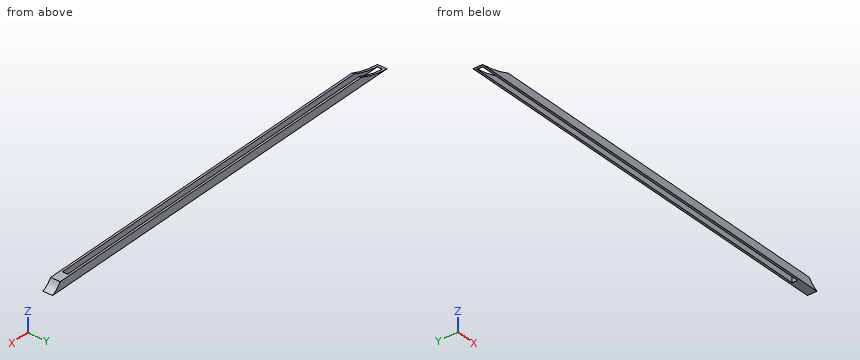
from build123d import *

# Parameters (mm, degrees)
SKETCH1_W               = 512.407402158
SKETCH1_H               = 11.43
SKETCH1_W_2             = 461.607402158
SKETCH1_H_2             = 6.35
BOSS_EXTRUDE1_DEPTH     = 9.652
CUT_EXTRUDE1_DEPTH      = 257.640102966
CUT_EXTRUDE1_DEPTH_BACK = 257.640102966
SKETCH2_R               = 121.331498574
SKETCH2_R_2             = 26.533992322


with BuildPart() as part:
    # Sketch1 → Boss-Extrude1 (new body)
    with BuildSketch(Plane.XY):
        Rectangle(SKETCH1_W, SKETCH1_H)
        Rectangle(SKETCH1_W_2, SKETCH1_H_2, mode=Mode.SUBTRACT)
    extrude(amount=BOSS_EXTRUDE1_DEPTH)

    # Sketch2 → Cut-Extrude1 (cut, two sides: drawn at the far end of the back side and taken through both)
    with BuildSketch(Plane(origin=(0, 5.715, 0), x_dir=(1, 0, 0), z_dir=(0, 1, 0)).offset(-CUT_EXTRUDE1_DEPTH_BACK)):
        with Locations((-245.184147657, -120.830054161)):
            Circle(SKETCH2_R)
        with Locations((267.338172934, -24.084772887)):
            Circle(SKETCH2_R_2)
    extrude(amount=CUT_EXTRUDE1_DEPTH + CUT_EXTRUDE1_DEPTH_BACK, mode=Mode.SUBTRACT)


solid = part.part
Verification items for the finished model (mm, model axes). Round coordinates to 2 decimals unless told otherwise and drop trailing zeros. Loops run counter-clockwise (first coordinate to the right, second up) from the corner with the lowest first, then second, coordinate; pieces in that order, holes last. Notation, with made-up numbers: (30.5, 51.5) - (57.5, 51.5) arc R21 cw to (57.5, 87.5) - close; hole circle Ø4 at (76, -17.5). An arc over 180 degrees is marked (long way). Answer in a Markdown table with one row per item. Add a question column.
Q1. Section check B-B on x = 209. Enter the section's corners in (y, z) (3 decimals).
Q2. Material ranges on line 1 (Y direction, x = 218, z = 5.75) (3 decimals); line 2 (X direction, y = 2, z = 6.75); line 3 (X direction, y = 0, z = 8.75), recorded low to high.
Q3. Section check A-A on y = 1.25. Enter the section's corners in (x, z), plus the area to 3 significant figures.
Q4. Section check C-C on z = 6.5. Enter the section's corners in (x, y) (3 decimals), plus the area to 3 significant figures.
Q5. Gauge pin test, flat ends, axial feed: pin 1 (5 mm diameter, centred on y = -0.5, z = 3, fed in from -X); pin 2 (5 mm diameter, centred on x = 167.5, y = 4.5, fed in from -Z); pin 3 (4 mm diameter, centred on x = -2.5, y = 1, fed in from +Z). Record the tip position at first contact, or that the pin passes through.
Found:
| question | item | result |
|---|---|---|
| 1 | outline | (-5.715, 0) - (-3.175, 0) - (-3.175, 9.652) - (-5.715, 9.652) - close; (3.175, 0) - (5.715, 0) - (5.715, 9.652) - (3.175, 9.652) - close |
| 2 | line 1 | y = -5.715 to -3.175, 3.175 to 5.715 |
| 2 | line 2 | x = 230.8 to 247.25 |
| 2 | line 3 | x = 230.8 to 245.68 |
| 3 | outline | (-234.16, 0) - (-230.8, 0) - (-230.8, 0.35) arc R121.33 cw to start; (230.8, 0) - (256.2, 0) arc R26.53 cw to (245.07, 9.65) - (230.8, 9.65) - close |
| 3 | area | 182 mm² |
| 4 | outline | (-204.564, -5.715) - (247.468, -5.715) - (247.468, 5.715) - (-204.564, 5.715) - (-204.564, 3.175) - (230.804, 3.175) - (230.804, -3.175) - (-204.564, -3.175) - close |
| 4 | area | 2,400 mm² |
| 5 | pin 1 | stops at x = 230.8 |
| 5 | pin 2 | stops at z = 0 |
| 5 | pin 3 | passes through |
